Geometry: see drawing. Coordinates: mm, zero at the bounding-box minimum. A direction names the side the tool comes from. Coordinates: 2 decimals unless noted, no trailing zeros. Write each loop counter-clockwise with the first axis right and the second up, starting at its lowest first coordinate (ties: lowest second). Pieces come first, ordered by that corner, then holes.
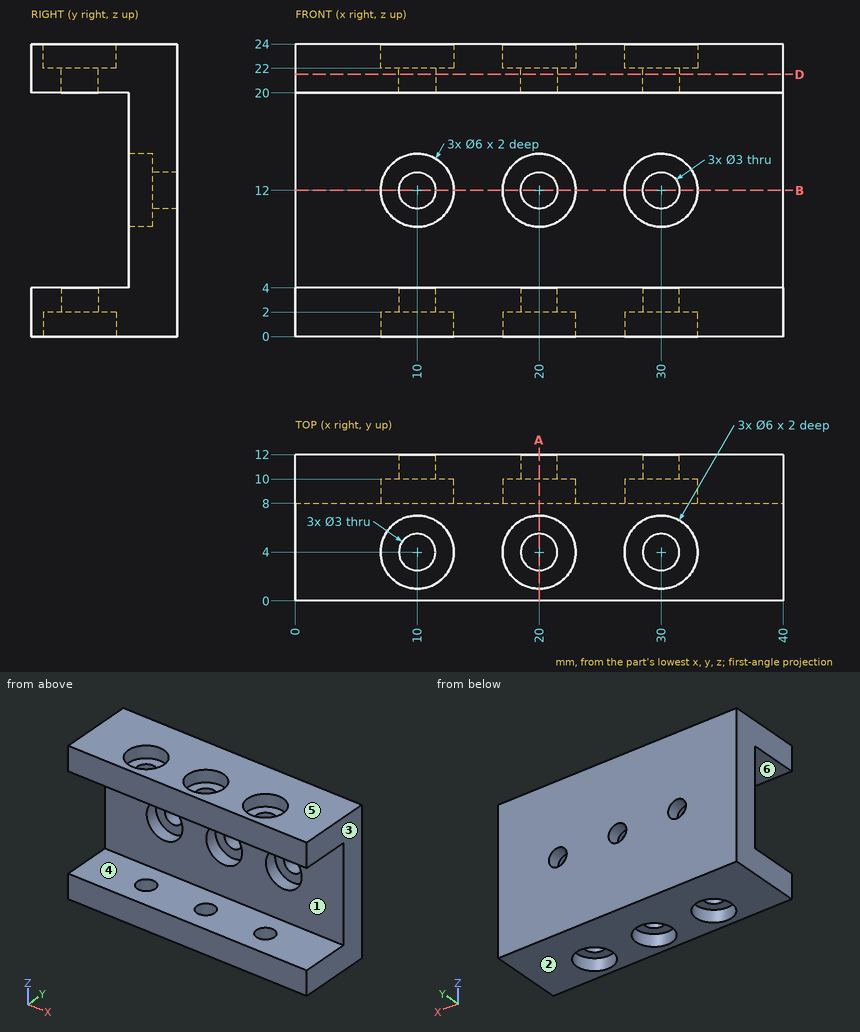
Item 1: Material intervals for probe 1 along X at (y, z) = (4, 23.35); probe 2 along X at (y, z) = (11.3, 12); probe 3 along Z at (x, y) = (36.5, 7), sorted ascending.
Derived:
probe 1: x = 0 to 7, 13 to 17, 23 to 27, 33 to 40
probe 2: x = 0 to 8.5, 11.5 to 18.5, 21.5 to 28.5, 31.5 to 40
probe 3: z = 0 to 4, 20 to 24
Item 2: Section A-A, the plane x = 20. State how many separate pieces and enclosed holes the cut face has, plus the area to 3 significant figures.
Derived:
separate pieces: 4
enclosed holes: 0
area: 106 mm2
Item 3: Section B-B, the plane z = 12. Output: boundary loops of the cut face in (x, y), plus the area to 3 significant figures.
Derived:
outline: (0, 8) - (7, 8) - (7, 10) - (8.5, 10) - (8.5, 12) - (0, 12) - close; (11.5, 10) - (13, 10) - (13, 8) - (17, 8) - (17, 10) - (18.5, 10) - (18.5, 12) - (11.5, 12) - close; (21.5, 10) - (23, 10) - (23, 8) - (27, 8) - (27, 10) - (28.5, 10) - (28.5, 12) - (21.5, 12) - close; (31.5, 10) - (33, 10) - (33, 8) - (40, 8) - (40, 12) - (31.5, 12) - close
area: 106 mm2
Item 4: Set-up query: the marked faces 1 and 2. Return all of +Z, -Z, +X, -X, +Y, -Y with unobstructed straight access to the full face (end or side cutting, diameter ignored); none if empty.
Derived:
face 1: +X, -X, -Y
face 2: -Z, +X, -X, +Y, -Y
Item 5: Section D-D, the plane z = 21.5. Output: boundary loops of the cut face in (x, y), plus the area to 3 significant figures.
Derived:
outline: (0, 0) - (40, 0) - (40, 12) - (0, 12) - close; hole circle Ø3 at (10, 4); hole circle Ø3 at (20, 4); hole circle Ø3 at (30, 4)
area: 459 mm2
Item 6: Pin query (flat end, axial travel): pin 1 (2.5 mm diameter, centred on x = 20, z = 12, fed in from -Y); pin 2 (4 mm diameter, centred on x = 23.5, y = 4.5, fed in from -Z); pin 3 (4 mm diameter, centred on x = 10, y = 4, fed in from -Z); pin 4 (4 mm diameter, centred on x = 10, y = 4, fed in from +Z). Return the tip coordinate at first contact, or that it passes through.
Derived:
pin 1: passes through
pin 2: stops at z = 0
pin 3: stops at z = 2
pin 4: stops at z = 22
Item 7: Pull-direction query (Z, two-part tool) for the marked faces 3, 4, 5 and 6; classes: released by +Z, released by -Z, zero draft, split by the parting line, or undercut.
Derived:
face 3: zero draft
face 4: undercut
face 5: released by +Z
face 6: undercut
